Source: CAD feature listing. Evaluate the final solid. Frame: model axes, mm. Give positions to 0.01 mm unless a question says otherwise; leave off trailing zeros. Write each loop counter-clockwise with the first axis right and the second up, starting at its lowest first coordinate (ties: lowest second). Pieces come first, ordered by that corner, then holes. Notation, with made-up numbers: M 30,-24 L 36,-24 A14 cw 36,-15 Z; hole C 80,88.5 d2. An arc over 180 degrees is marked long. Answer as a JSON object with one key per item and string values. Group by question number.
```python
from build123d import *

# Parameters (mm, degrees)
BOSS_EXTRUDE1_DEPTH = 434.6
FILLET1_R           = 25.4
FILLET2_R           = 12.7


with BuildPart() as part:
    # Sketch1 → Boss-Extrude1 (new body)
    with BuildSketch(Plane.XY):
        with BuildLine():
            Line((-50.8, 241.861797239), (-50.8, 190.955582052))
            ThreePointArc((-50.8, 190.955582052), (-248.54641158, 223.033274611), (-436.283591965, 292.943021812))
            Line((-436.283591965, 292.943021812), (-413.99080623, 338.590274786))
            ThreePointArc((-413.99080623, 338.590274786), (-237.101828879, 272.554605518), (-50.8, 241.861797239))
        make_face()
    extrude(amount=-BOSS_EXTRUDE1_DEPTH)

    # Fillet1
    fillet1_edges = [part.edges().sort_by_distance(p)[0] for p in [
        (-425.137199097, 315.766648299, -434.6),
        (-425.137199097, 315.766648299, 0),
    ]]
    fillet(fillet1_edges, radius=FILLET1_R)

    # Fillet2
    fillet2_edges = [part.edges().sort_by_distance(p)[0] for p in [
        (-236.247784218, 219.860784348, -434.6),
        (-236.247784218, 219.860784348, 0),
        (-436.283591965, 292.943021812, -217.3),
        (-429.586107636, 289.70220341, -427.161351846),
        (-429.586107636, 289.70220341, -7.438648154),
        (-413.99080623, 338.590274786, -217.3),
        (-224.807276662, 269.365840187, -434.6),
        (-407.292621944, 335.350680861, -427.161443503),
        (-407.292621944, 335.350680861, -7.438556497),
        (-224.807276662, 269.365840187, 0),
    ]]
    fillet(fillet2_edges, radius=FILLET2_R)


solid = part.part
```
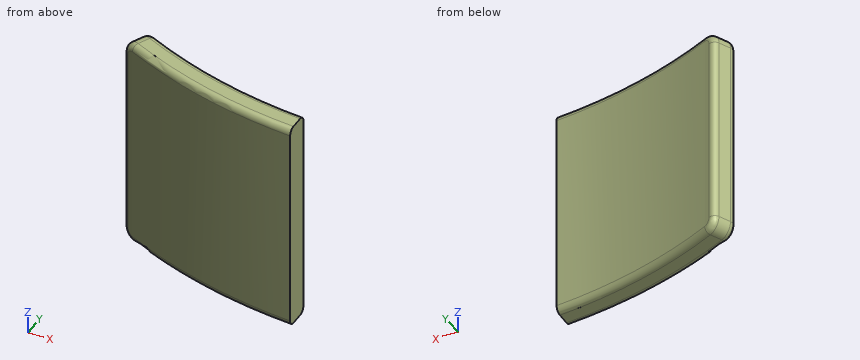
(1) Ray query, L1, parallel to Y at x = -342.5, z = -343; L2, parallel to X at y = 307, z = -222; L3, parallel to Y at x = -285.5, z = -313.5. Return the intervals inside material, ascending. Write a range as [from, to].
(2) Contact query for flat-ended pins moving along their axis: pin 1 Ø6 at (x, z) = (-351.5, -281) entering from +Y; pin 2 Ø5 at (x, y) = (-373.5, 310) entering from -Z; pin 3 Ø1.5 at (x, z) = (-107.5, -136.5) entering from +Y. Output: stop coordinate, or through.
(3) Section A-A, the plane z = -39. Return loops of the section in (x, y) (3 decimals), plus the area to 3 significant figures.
Reported:
{
 "1": {"L1": "y = [252.79, 307.16]", "L2": "x = [-429.42, -342.1]", "L3": "y = [233.55, 286.8]"},
 "2": {"pin 1": "stops at y = 311.96", "pin 2": "stops at z = -434.56", "pin 3": "stops at y = 247.39"},
 "3": {"outline": "M -430.675,304.426 A12.7 ccw -424.693,287.372 A1025.525 ccw -50.8,190.956 L -50.8,241.862 A974.725 cw -402.69,333.161 A12.7 ccw -419.528,327.252 Z", "area": "19,700 mm2"}
}
